CAD build for the part. Positions are in the model's coordinates, mm. Face numbers are marked on the shaded views. A direction names the side the tool comes from. Round coordinates to 2 decimals unless told otherwise and drop trailing zeros. Write each loop counter-clockwise with the first axis right and the second up, starting at its lowest first coordinate (ties: lowest second). Pieces come first, ordered by that corner, then holes. Notation, with made-up numbers: (1, -17) - (55, -17) arc R25 cw to (55, 8) - close; hole circle Ø6 at (41.5, 58). An arc over 180 degrees is marked (long way). Put each result on its own line as item: value. Start each with the question number.
Item 1: Mould opens along Y. For the marked faces 6, 7, 8 and 9 say: released by +Y, released by -Y, zero draft, split by the parting line, or undercut.
Item 2: Cut at D-D (z = 15.5). Give the cut face in (x, y), and give its area (3 significant figures).
Item 3: Cut at A-A (x = 15). Give the cut face in (y, z), and give its area (3 significant figures).
Item 4: 3-axis set-ups, long thin cutter, end or side, ignore diameter. For the marked faces 1, 2, 3, 4 and 5: which of +Z, -Z, +X, -X, +Y, -Y reach the whole face in a straight line?
Item 5: Pin check, flat tips, straight feed: pin 1 Ø4 at (y, z) = (-11, 0.5) entering from +X; pin 2 Ø12 at (x, z) = (-0.5, 14.5) entering from +Y; pin 3 Ø10 at (x, z) = (13.5, 11.5) entering from -Y. Stop position of each tip, or through.
Item 6: Drill centre lines: line 1 (X direction, y = -15, z = -0.65); line 2 (X direction, y = -7.5, z = 0.75); line 3 (X direction, y = 7.5, z = 5). Where is each one in solid material? Low to high. Write a range as from..to.
Item 7: Cut at B-B (y = -9). Give the cut face in (x, z), and give its area (3 significant figures).
Item 8: Cut at C-C (z = 0.5). Give the cut face in (x, y).
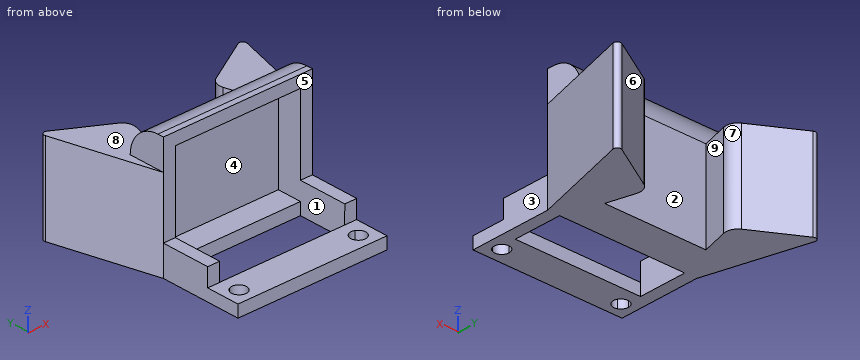
```python
from build123d import *

# Parameters (mm, degrees)
BOSS_EXTRUDE1_DEPTH  = 16
SKETCH3_W            = 25
SKETCH3_H            = 6
BOSS_EXTRUDE2_DEPTH  = 2
SKETCH6_W            = 25
SKETCH6_H            = 15
BOSS_EXTRUDE3_DEPTH  = 2
SKETCH7_W            = 21
SKETCH7_H            = 8
CUT_EXTRUDE1_DEPTH   = 2
SKETCH10_W           = 25
SKETCH10_H           = 4.5
BOSS_EXTRUDE4_DEPTH  = 2
CUT_EXTRUDE2_DEPTH   = 3
FILLET1_R            = 5
BOSS_EXTRUDE7_DEPTH  = 15
BOSS_EXTRUDE8_DEPTH  = 2
BOSS_EXTRUDE9_DEPTH  = 2
FILLET4_R            = 2
FILLET5_R            = 0.6
SKETCH16_W           = 3
SKETCH16_H           = 8.020078622
BOSS_EXTRUDE10_DEPTH = 2
BOSS_EXTRUDE11_DEPTH = 2
SKETCH18_W           = 21
SKETCH18_H           = 13
CUT_EXTRUDE3_DEPTH   = 4


with BuildPart() as part:
    # Sketch1 → Boss-Extrude1 (new body)
    with BuildSketch(Plane.XY):
        Polygon((23, 2), (-2, 2), (-2, -4), (0, -4), (0, 0), (21, 0), (21, -4), (23, -4), align=None)
    extrude(amount=BOSS_EXTRUDE1_DEPTH)

    # Sketch3 → Boss-Extrude2 (add)
    with BuildSketch(Plane.XY.offset(16)):
        with Locations((10.5, -1)):
            Rectangle(SKETCH3_W, SKETCH3_H)
    extrude(amount=BOSS_EXTRUDE2_DEPTH)

    # Sketch6 → Boss-Extrude3 (add)
    with BuildSketch(Plane(origin=(0, 0, 0), x_dir=(-1, 0, 0), z_dir=(0, 0, -1))):
        with Locations((-10.5, -5.5)):
            Rectangle(SKETCH6_W, SKETCH6_H)
    extrude(amount=BOSS_EXTRUDE3_DEPTH)

    # Sketch7 → Cut-Extrude1 (cut)
    with BuildSketch(Plane(origin=(0, 0, -2), x_dir=(-1, 0, 0), z_dir=(0, 0, -1))):
        with Locations((-10.5, -8)):
            Rectangle(SKETCH7_W, SKETCH7_H)
    extrude(amount=-CUT_EXTRUDE1_DEPTH, mode=Mode.SUBTRACT)

    # Sketch10 → Boss-Extrude4 (add)
    with BuildSketch(Plane(origin=(0, 0, -2), x_dir=(-1, 0, 0), z_dir=(0, 0, -1))):
        with Locations((-10.5, -15.25)):
            Rectangle(SKETCH10_W, SKETCH10_H)
    extrude(amount=-BOSS_EXTRUDE4_DEPTH)

    # Sketch11 → Cut-Extrude2 (cut)
    with BuildSketch(Plane(origin=(0, 0, -2), x_dir=(-1, 0, 0), z_dir=(0, 0, -1))):
        with BuildLine():
            ThreePointArc((-19.246874512, -15), (-19.813649388, -13.953241465), (-21, -13.855725233))
            Line((-21, -13.855725233), (-21, -16.144274767))
            ThreePointArc((-21, -16.144274767), (-19.813649388, -16.046758535), (-19.246874512, -15))
        make_face()
        with BuildLine():
            Line((-21, -16.144274767), (-21, -13.855725233))
            ThreePointArc((-21, -13.855725233), (-21.746874512, -15), (-21, -16.144274767))
        make_face()
        with BuildLine():
            ThreePointArc((0.753125488, -15), (0.548016186, -14.313921703), (0, -13.852997071))
            Line((0, -13.852997071), (0, -16.147002929))
            ThreePointArc((0, -16.147002929), (0.548016186, -15.686078297), (0.753125488, -15))
        make_face()
        with BuildLine():
            Line((0, -16.147002929), (0, -13.852997071))
            ThreePointArc((0, -13.852997071), (-1.746874512, -15), (0, -16.147002929))
        make_face()
    extrude(amount=-CUT_EXTRUDE2_DEPTH, mode=Mode.SUBTRACT)

    # Fillet1
    fillet1_edges = [part.edges().sort_by_distance(p)[0] for p in [
        (10.5, 2, 18),
    ]]
    fillet(fillet1_edges, radius=FILLET1_R)

    # Sketch13 → Boss-Extrude7 (add)
    with BuildSketch(Plane(origin=(0, 0, -2), x_dir=(-1, 0, 0), z_dir=(0, 0, -1))):
        Polygon((-21, -4), (-23, -4), (-27.823085464, 14), (-17.406964655, 8.041440838), (-19, 2), (-2, 2), (-3.607695155, 8), (6.784609691, 14), (2, -4), (0, -4), align=None)
        Polygon((-22.232673012, -3), (-26.235818051, 11.939940677), (-18.569558802, 7.554444375), (-20.297865317, 1), (-0.696774627, 1), (-2.44317049, 7.51763809), (5.199725285, 11.930266023), (1.231086646, -3), (0, -3), (-21, -3), align=None, mode=Mode.SUBTRACT)
    extrude(amount=-BOSS_EXTRUDE7_DEPTH)

    # Sketch14 → Boss-Extrude8 (add)
    with BuildSketch(Plane(origin=(0, 0, -2), x_dir=(-1, 0, 0), z_dir=(0, 0, -1))):
        Polygon((-27.823085464, 14), (-23, -4), (-19, 2), (-17.406964655, 8.041440838), align=None)
        Polygon((-2, 2), (2, -4), (6.784609691, 14), (-3.607695155, 8), align=None)
    extrude(amount=-BOSS_EXTRUDE8_DEPTH)

    # Sketch15 → Boss-Extrude9 (add)
    with BuildSketch(Plane.XY.offset(13)):
        Polygon((-6.784609691, 14), (-2, -4), (2, 2), (3.607695155, 8), align=None)
        Polygon((19, 2), (23, -4), (27.823085464, 14), (17.406964655, 8.041440838), align=None)
    extrude(amount=-BOSS_EXTRUDE9_DEPTH)

    # Fillet4
    fillet4_edges = [part.edges().sort_by_distance(p)[0] for p in [
        (17.406964655, 8.041440838, 5.5),
        (3.607695155, 8, 5.5),
    ]]
    fillet(fillet4_edges, radius=FILLET4_R)

    # Fillet5
    fillet5_edges = [part.edges().sort_by_distance(p)[0] for p in [
        (27.823085464, 14, 5.5),
        (-6.784609691, 14, 5.5),
    ]]
    fillet(fillet5_edges, radius=FILLET5_R)

    # Sketch16 → Boss-Extrude10 (add)
    with BuildSketch(Plane.ZY.offset(2)):
        with Locations((1.5, -8.010039311)):
            Rectangle(SKETCH16_W, SKETCH16_H)
    extrude(amount=-BOSS_EXTRUDE10_DEPTH)

    # Sketch17 → Boss-Extrude11 (add)
    with BuildSketch(Plane(origin=(23, 0, 0), x_dir=(0, 0, -1), z_dir=(1, 0, 0))):
        Polygon((0, -12), (-3, -12.020078622), (-3, -4), (0, -4), align=None)
    extrude(amount=-BOSS_EXTRUDE11_DEPTH)

    # Sketch18 → Cut-Extrude3 (cut)
    with BuildSketch(Plane.XZ.offset(4)):
        with Locations((10.5, 6.5)):
            Rectangle(SKETCH18_W, SKETCH18_H)
    extrude(amount=-CUT_EXTRUDE3_DEPTH, mode=Mode.SUBTRACT)


solid = part.part
```
Output values:
1. face 6: released by +Y
1. face 7: undercut
1. face 8: zero draft
1. face 9: undercut
2. outline: (-2, -4) - (0, -4) - (0, 0) - (21, 0) - (21, -4) - (23, -4) - (23, 1.33) - (-2, 1.33) - close
2. area: 49.3 mm2
3. outline: (-17.5, -2) - (-12, -2) - (-12, 0) - (-17.5, 0) - close; (-4, -2) - (2, -2) - (2, 13) arc R5 ccw to (-3, 18) - (-4, 18) - (-4, 16) - (0, 16) - (0, 0) - (-4, 0) - close
3. area: 61.6 mm2
4. face 1: none
4. face 2: +Z, -Z
4. face 3: +Z, -Z, +X, -Y
4. face 4: -Y
4. face 5: +Z, +X, -X, -Y
5. pin 1: x = 23
5. pin 2: y = 13.36
5. pin 3: y = -4
6. line 1: -2..-0.75, 1.75..19.25, 21.75..23
6. line 2: -2..0, 21..23
6. line 3: -5.06..-4.02, 2.44..3.22, 17.78..18.58, 25.05..26.08
7. outline: (-2, -2) - (0, -2) - (0, 3) - (-2, 3) - close; (21, -2) - (23, -2) - (23, 3) - (21, 3) - close
7. area: 20.0 mm2
8. outline: (-6.41, 12.6) - (-2, -4) - (-2, -12.02) - (0, -12.02) - (0, 0) - (21, 0) - (21, -12) - (23, -12) - (23, -4) - (27.45, 12.61) arc R0.6 ccw to (26.57, 13.28) - (18.74, 8.8) arc R2 ccw to (17.8, 6.56) - (19, 2) - (2, 2) - (3.21, 6.52) arc R2 ccw to (2.28, 8.77) - (-5.53, 13.28) arc R0.6 ccw to start; hole (-5.2, 11.93) - (-2, -0.11) - (-2, 2) - (0.96, 2) - (2.44, 7.52) - close; hole (18.57, 7.55) - (20.03, 2) - (23, 2) - (23, -0.14) - (26.24, 11.94) - close
